Here's how the part is built. I have some questions about the finished solid (model axes, mm). A direction names the side the tool comes from. Coordinates: 2 decimals unless noted, no trailing zeros. Loops run counter-clockwise (first coordinate to the right, second up) from the corner with the lowest first, then second, coordinate; pieces in that order, holes last.
```python
from build123d import *

# Parameters (mm, degrees)
SKETCH_1_W          = 6
SKETCH_1_H          = 26
SKETCH_1_R          = 1.6
EXTRUDE_1_DEPTH     = 3
EXTRUDE_1_2_DEPTH   = 3
SKETCH_11_W         = 3
SKETCH_11_H         = 10
SKETCH_10_W         = 3
SKETCH_10_H         = 26
SKETCH_13_W         = 3
SKETCH_13_H         = 10
SKETCH_12_W         = 3
SKETCH_12_H         = 26
SKETCH_14_W         = 50
SKETCH_14_H         = 10
EXTRUDE_4_DEPTH     = 3
SKETCH_15_W         = 19.024799208
SKETCH_15_H         = 22.305451654
CUT_EXTRUDE_2_DEPTH = 3
SKETCH_16_W         = 14.351226191
SKETCH_16_H         = 17.437681629
CUT_EXTRUDE_3_DEPTH = 3
SKETCH_17_W         = 3
SKETCH_17_H         = 26
EXTRUDE_5_DEPTH     = 3
EXTRUDE_6_DEPTH     = 3
EXTRUDE_10_DEPTH    = 2.961896
EXTRUDE_11_DEPTH    = 2.961896
CUT_EXTRUDE_4_DEPTH = 100
SKETCH_22_W         = 3
SKETCH_22_H         = 51.402298851
EXTRUDE_12_DEPTH    = 3
CUT_EXTRUDE_5_DEPTH = 3
SKETCH_24_R         = 0.7
CUT_EXTRUDE_6_DEPTH = 10


with BuildPart() as part:
    # Sketch 1 → Extrude 1 (new body)
    with BuildSketch(Plane(origin=(0, 0, 0), x_dir=(0, 0, -1), z_dir=(1, 0, 0))):
        with Locations((-2.817174515, -6.083780501)):
            Rectangle(SKETCH_1_W, SKETCH_1_H)
        with Locations((-2.817174515, -16.083780501)):
            Circle(SKETCH_1_R, mode=Mode.SUBTRACT)
        with Locations((-2.817174515, 3.916219499)):
            Circle(SKETCH_1_R, mode=Mode.SUBTRACT)
    extrude(amount=EXTRUDE_1_DEPTH)



with BuildPart() as body_2:
    # Sketch 1 → Extrude 1 2 (new body)
    with BuildSketch(Plane(origin=(0, 0, 0), x_dir=(0, 0, -1), z_dir=(1, 0, 0))):
        with Locations((-86.817174515, -6.083780501)):
            Rectangle(SKETCH_1_W, SKETCH_1_H)
        with Locations((-86.817174515, -16.083780501)):
            Circle(SKETCH_1_R, mode=Mode.SUBTRACT)
        with Locations((-86.817174515, 3.916219499)):
            Circle(SKETCH_1_R, mode=Mode.SUBTRACT)
    extrude(amount=EXTRUDE_1_2_DEPTH)


with BuildPart() as body_3:
    # Sketch 11 → Loft 4 section 0
    with BuildSketch(Plane.ZY.offset(-90)):
        with Locations((21.317174515, 13.916219499)):
            Rectangle(SKETCH_11_W, SKETCH_11_H)
    # Sketch 10 → Loft 4 section 1
    with BuildSketch(Plane(origin=(3, 0, 0), x_dir=(0, 0, -1), z_dir=(1, 0, 0))):
        with Locations((-7.317174515, -6.083780501)):
            Rectangle(SKETCH_10_W, SKETCH_10_H)
    loft()



with BuildPart() as body_4:
    # Sketch 13 → Loft 5 section 0
    with BuildSketch(Plane.ZY.offset(-90)):
        with Locations((68.317174515, 13.916219499)):
            Rectangle(SKETCH_13_W, SKETCH_13_H)
    # Sketch 12 → Loft 5 section 1
    with BuildSketch(Plane(origin=(3, 0, 0), x_dir=(0, 0, -1), z_dir=(1, 0, 0))):
        with Locations((-82.317174515, -6.083780501)):
            Rectangle(SKETCH_12_W, SKETCH_12_H)
    loft()


with BuildPart() as body_3_1:
    add(body_3.part)

    add(body_4.part)  # Extrude 4 merges body 4
    # Sketch 14 → Extrude 4 (add)
    with BuildSketch(Plane(origin=(90, 0, 0), x_dir=(0, 0, -1), z_dir=(1, 0, 0))):
        with Locations((-44.817174515, 13.916219499)):
            Rectangle(SKETCH_14_W, SKETCH_14_H)
    extrude(amount=EXTRUDE_4_DEPTH)

    # Sketch 15 → Cut-Extrude 2 (cut)
    with BuildSketch(Plane(origin=(13.223093182, 0, 82.172079061), x_dir=(0.987298603, 0, -0.158875637), z_dir=(0.158875637, 0, 0.987298603))):
        with Locations((78.439469875, 13.430311671)):
            Rectangle(SKETCH_15_W, SKETCH_15_H)
    extrude(amount=CUT_EXTRUDE_2_DEPTH, mode=Mode.SUBTRACT)

    # Sketch 16 → Cut-Extrude 3 (cut)
    with BuildSketch(Plane(origin=(-0.83674418, 0, 5.199767406), x_dir=(-0.987298603, 0, -0.158875637), z_dir=(0.158875637, 0, -0.987298603))):
        with Locations((-93.553254701, 14.072952005)):
            Rectangle(SKETCH_16_W, SKETCH_16_H)
    extrude(amount=CUT_EXTRUDE_3_DEPTH, mode=Mode.SUBTRACT)


with BuildPart() as part_1:
    add(part.part)

    add(body_2.part)  # Extrude 5 merges body 2

    add(body_3_1.part)  # Extrude 5 merges body 3
    # Sketch 17 → Extrude 5 (add)
    with BuildSketch(Plane.ZY.offset(-3)):
        with Locations((7.317174515, -6.083780501)):
            Rectangle(SKETCH_17_W, SKETCH_17_H)
        with Locations((82.317174515, -6.083780501)):
            Rectangle(SKETCH_17_W, SKETCH_17_H)
    extrude(amount=EXTRUDE_5_DEPTH)

    # Sketch 18 → Extrude 6 (add)
    with BuildSketch(Plane(origin=(0, 18.916219499, 0), x_dir=(1, 0, 0), z_dir=(0, 1, 0))):
        Polygon((93, -69.334415895), (67, -73.518323941), (67, -16.11602509), (93, -20.299933136), align=None)
    extrude(amount=-EXTRUDE_6_DEPTH)

    # Sketch 19 → Extrude 10 (add)
    with BuildSketch(Plane(origin=(13.223093182, 0, 82.172079061), x_dir=(0.987298603, 0, -0.158875637), z_dir=(0.158875637, 0, 0.987298603))):
        Polygon((-10.354611208, 6.916219499), (54.468735845, 18.916219499), (57.643062592, 15.200587801), (10.872988387, 4.084352126), align=None)
    extrude(amount=-EXTRUDE_10_DEPTH)

    # Sketch 20 → Extrude 11 (add)
    with BuildSketch(Plane(origin=(-0.83674418, 0, 5.199767406), x_dir=(-0.987298603, 0, -0.158875637), z_dir=(0.158875637, 0, -0.987298603))):
        Polygon((-3.886103118, 6.916219499), (-68.709450171, 18.916219499), (-71.52946793, 14.93833866), (-30.165426117, 5.801086138), align=None)
    extrude(amount=-EXTRUDE_11_DEPTH)

    # Sketch 21 → Cut-Extrude 4 (cut)
    with BuildSketch(Plane(origin=(0, 0, -0.182825485), x_dir=(-1, 0, 0), z_dir=(0, 0, -1))):
        Polygon((-3, -19.083780501), (-93, 13.916219499), (-93, 8.916219499), align=None)
    extrude(amount=-CUT_EXTRUDE_4_DEPTH, mode=Mode.SUBTRACT)

    # Sketch 22 → Extrude 12 (add)
    with BuildSketch(Plane.XZ.offset(-15.916219499)):
        with Locations((68.5, 44.817174515)):
            Rectangle(SKETCH_22_W, SKETCH_22_H)
    extrude(amount=EXTRUDE_12_DEPTH)

    # Sketch 23 → Cut-Extrude 5 (cut)
    with BuildSketch(Plane(origin=(70, 0, 0), x_dir=(0, 0, -1), z_dir=(1, 0, 0))):
        with BuildLine():
            Line((-19.598783711, 12.916219499), (-70.03556532, 12.916219499))
            ThreePointArc((-70.03556532, 12.916219499), (-44.817174515, 15.916219499), (-19.598783711, 12.916219499))
        make_face()
    extrude(amount=-CUT_EXTRUDE_5_DEPTH, mode=Mode.SUBTRACT)

    # Sketch 24 → Cut-Extrude 6 (cut)
    with BuildSketch(Plane(origin=(0, 18.916219499, 0), x_dir=(1, 0, 0), z_dir=(0, 1, 0))):
        with Locations((89.1, -67.417174515)):
            Circle(SKETCH_24_R)
        with Locations((71.1, -67.417174515)):
            Circle(SKETCH_24_R)
        with Locations((71.1, -22.217174515)):
            Circle(SKETCH_24_R)
        with Locations((89.1, -22.217174515)):
            Circle(SKETCH_24_R)
    extrude(amount=-CUT_EXTRUDE_6_DEPTH, mode=Mode.SUBTRACT)


solid = part_1.part
```
1. I need wall thicknesses on line 1 along Z through (x, y) = (71, 17); line 2 along X through (y, z) = (17.5, 66.5); line 3 along Y through (x, z) = (79.5, 23.5). Which ranges of each line are inside material? Lowest first, please.
2. I want a section at D-D (z = 62.5). Please give me the cut outline in (x, y), then the cut area to 3 significant figures.
3. I want a section at B-B (x = 45). Please give me the cut outline in (y, z), then the cut area to 3 significant figures.
4. I want a section at A-A (x = 14). Please give me the cut outline in (y, z).
5. We'd pull the mould along X, two halves only. Please class faces 6 (the flat face through (2, -6, 8.817)), 7 (the flat face through (93, 16, 45)), 8 (the flat face through (70, 15, 64)), 9 (the flat face through (90, 14, 45)): +X half, -X half, draft (parallel to the pull), parting line (faces both ways), or undercut.
6. On a 3-axis mill with a long thin cutter (end or side, diameter ignored), from which of +Z, -Z, +X, -X, +Y, -Y can I reach the whole of each face in a straight line? I mean faces 1 (the flat face through (44.466, 13.389, 74.144)), 2 (the flat face through (0, -6, 85)), 3 (the cylindrical face through (68.521, 15.916, 45.174)), 4 (the flat face through (3, -6, 87)), 5 (the flat face through (70, 15, 26)). Say none if no direction works.
7. I want a section at C-C (z = 53). Please give me the cut outline in (x, y), then the cut area to 3 significant figures.
8. For pin 1 (1.5 mm diameter, centred on y = -4, z = 16.5, fed in from -X); pin 2 (5 mm diameter, centred on y = 15, z = 39, fed in from -X); pin 3 (0.5 mm diameter, centred on x = 69, z = 70.5, fed in from -Y); pin 4 (5 mm diameter, centred on x = 27, y = -12.5, fed in from -Z), each with a flat end and sliding along its axis, tell me the tip position at first contact or that it passes through.
Response values:
1. line 1: z = 16.76 to 21.52, 22.91 to 66.72, 68.11 to 72.87
1. line 2: x = 67 to 93
1. line 3: y = 15.92 to 18.92
2. outline: (67, 14.45) - (70, 14.45) - (70, 15.92) - (90, 15.92) - (90, 12.82) - (93, 13.92) - (93, 18.92) - (67, 18.92) - close
2. area: 90.0 mm2
3. outline: (-3.68, 12.58) - (14.79, 12.58) - (14.88, 15.58) - (-3.68, 15.58) - close; (-3.68, 74.06) - (14.88, 74.06) - (14.79, 77.06) - (-3.68, 77.06) - close
3. area: 111 mm2
4. outline: (-15.05, 7.59) - (8.98, 7.59) - (9.07, 10.59) - (-15.05, 10.59) - close; (-15.05, 79.05) - (9.07, 79.05) - (8.98, 82.05) - (-15.05, 82.05) - close
5. face 6: draft
5. face 7: +X half
5. face 8: undercut
5. face 9: undercut
6. face 1: -X, +Y, -Y
6. face 2: +Z, -Z, -X, +Y, -Y
6. face 3: -X, -Y
6. face 4: +Z, +X, +Y, -Y
6. face 5: -Y
7. outline: (67, 15.6) - (70, 15.6) - (70, 15.92) - (90, 15.92) - (90, 12.82) - (93, 13.92) - (93, 18.92) - (67, 18.92) - close
7. area: 86.6 mm2
8. pin 1: passes through
8. pin 2: stops at x = 67
8. pin 3: stops at y = 5.02
8. pin 4: stops at z = 9.35
